Design review of the part built by this model. Coordinates are the model's own, in mm. Give positions to 0.01 mm unless a question says otherwise; leave off trailing zeros. Write each loop counter-clockwise with the first axis right and the second up, starting at its lowest first coordinate (ties: lowest second). Pieces come first, ordered by that corner, then holes. Notation, with made-up numbers: (-14, 52) -> (41, 52) arc R18 ccw to (41, 56) -> close; hole circle Ø8 at (41.5, -13). An arc over 180 degrees is marked (long way). Answer as a JSON object with one key per item and string values.
Autodesk Inventor part; units mm, degrees
ref_plane "nut_XY" through (0, 0, 1.0033) normal (0, 0, 1) x (1, 0, 0)
ref_plane "nut_YZ" through (0, 0, 1.0033) normal (1, 0, 0) x (0, 1, 0)
ref_plane "nut_ZX" through (0, 0, 1.0033) normal (0, 1, 0) x (0, 0, 1)
sketch "Sketch_1" plane through (0, 0, 0) normal (1, 0, 0) x (0, 1, 0)
  line L0 (0, -1.0033) -> (0, 1.0033)
  line L1 (0, 1.0033) -> (6.9977, 1.0033)
  line L2 (6.9977, 1.0033) -> (8.3972, 0.4939)
  line L3 (8.3972, 0.4939) -> (8.3972, -0.4939)
  line L4 (8.3972, -0.4939) -> (6.9977, -1.0033)
  line L5 (6.9977, -1.0033) -> (0, -1.0033)
  line L6 (0, -1.0033) -> (0, 1.0033)
revolve "Revolution1" add sketch "Sketch_1" angle 360 about axis through (0, 0, -1.0033) along (0, 0, -1)
sketch "Sketch_2" plane through (0, 0, 0) normal (0, 0, 1) x (1, 0, 0)
  line L0 (-13.9954, 13.9954) -> (-13.9954, -13.9954)
  line L1 (-13.9954, -13.9954) -> (13.9954, -13.9954)
  line L2 (13.9954, -13.9954) -> (13.9954, 13.9954)
  line L3 (13.9954, 13.9954) -> (-13.9954, 13.9954)
  line L4 (-8.001, 0) -> (-4.0401, -6.9977)
  line L5 (-4.0401, -6.9977) -> (4.0401, -6.9977)
  line L6 (4.0401, -6.9977) -> (8.001, 0)
  line L7 (8.001, 0) -> (4.0401, 6.9977)
  line L8 (4.0401, 6.9977) -> (-4.0401, 6.9977)
  line L9 (-4.0401, 6.9977) -> (-8.001, 0)
extrude "Extrusion1" cut sketch "Sketch_2" along normal mid plane 4.0132
sketch "Sketch3" plane through (0, 0, -1.0033) normal (0, 0, -1) x (-1, 0, 0)
  point P0 (0, 0)
hole "Drilling 1" at (0, 0, -1.0033) direction (0, 0, 1) diameter 10.106 depth 2.0066 countersink diameter 11.9888 countersink angle 90
ref_plane "nut_XY" through (0, 0, 1.0033) normal (0, 0, 1) x (1, 0, 0)
ref_plane "nut_YZ" through (0, 0, 1.0033) normal (1, 0, 0) x (0, 1, 0)
ref_plane "nut_ZX" through (0, 0, 1.0033) normal (0, 1, 0) x (0, 0, 1)
properties part number "AT527M"
(1) The part is to be moulded in two halves that separate along Y. For faces 1 (the conical face through (-3.53, 6.3, -0.92)), 2 (the conical face through (7.242, 0.014, 0.915)), 3 (the cylindrical face through (3.075, -4.01, 0.478)), 4 (the flat face through (5.99, -3.55, -0.01)), say which applies: +Y half, -Y half, draft (parallel to the pull), parting line (faces both ways), or undercut.
Here are the results:
{"face 1": "+Y half", "face 2": "parting line", "face 3": "undercut", "face 4": "-Y half"}
(2) We need section A-A, the plane z = -0.4. State the section outline as (x, y) points.
Here are the results:
{"outline": "(-8, 0) -> (-4.04, -7) -> (4.04, -7) -> (8, 0) -> (4.04, 7) -> (-4.04, 7) -> close; hole circle Ø10.78 at (0, 0)"}
(3) Clearance check with a flat-ended pin moving along its axis: pin 1 (1.5 mm diameter, centred on x = -4, y = -3, fed in from -Z). State where the tip first meets the part, or that it passes through.
Here are the results:
{"pin 1": "stops at z = -0.76"}
(4) For line 1 along Y through (x, z) = (0, 0.2); line 2 along X through (y, z) = (1.75, 0.85); line 3 along X through (y, z) = (-3.5, 0.3), list the stretches that pass through material, from the lowest coordinate up.
Here are the results:
{"line 1": "y = -7 to -5.05, 5.05 to 7", "line 2": "x = -7.01 to -4.74, 4.74 to 7.01", "line 3": "x = -6.02 to -3.64, 3.64 to 6.02"}
